The listing builds one solid part. Answer for the finished solid, in the listing's coordinates (mm). A direction names the side the tool comes from. Round coordinates to 2 decimals unless told otherwise and drop trailing zeros. Order: outer loops, then holes, each group sorted by start corner. A loop starts at its lowest first (then second) coordinate and runs counter-clockwise, first axis right, second up. Notation, with made-up numbers: M 63,70.5 L 100,70.5 A31 cw 100,109.5 Z; hole C 23.25,-1 d3. An arc over 180 degrees is marked long. Write item = value, one per line. Start each with the question number.
(1) For a pull along Z with two mould halves and no side action, classify faces 6 (the face through (-2, 58, -50)), 7 (the face through (-2.573, 119.082, -87.102)), 8 (the face through (-59.63, 23, 15)) as released by +Z, released by -Z, zero draft, split by the parting line, or undercut.
(2) Straight lines are drawn through the part: probe 1 along Z at (x, y) = (-1.5, 90.5); probe 2 along Y at (x, z) = (9, -2); probe 3 along X at (y, z) = (82, -42.5). For each, find the intervals that lie inside material, in ascending order. Write a range as from..to.
(3) Which of the six approach directions +Z, -Z, +X, -X, +Y, -Y give full straight-line access (tool end or side, diameter ignored) to faces 1 (the face through (-3, 43.505, 6)), 2 (the face through (17.87, 59, -34)), 3 (the face through (-2.57, 124, -80.01)), 4 (the face through (-33, 28, 0)), 5 (the face through (-2, 113.505, -80))?
(4) A cutting plane is placed at D-D, the plane x = 6. Determine the outline of the cut face in (y, z).
(5) Each of these flat-tipped pins is pushed along its axis until it touches: pin 1 (12 mm diameter, centred on x = 7, z = -63, fed in from +Y); pin 2 (8 mm diameter, centred on x = -1.05, z = -85.12, fed in from -Y); pin 3 (11 mm diameter, centred on x = -38.5, y = 28, fed in from -Z). Where does it stop, or does it pass through?
(6) A cutting plane is placed at C-C, the plane z = -98. Determine the outline of the cut face in (x, y).
(7) A cutting plane is placed at B-B, the plane y = 16.5. Determine the outline of the cut face in (x, z).
(8) A cutting plane is placed at A-A, the plane z = 12. Determine the outline of the cut face in (x, y), and give its area (3 significant figures).
from build123d import *

# Parameters (mm, degrees)
SKETCH2_W           = 115
SKETCH2_H           = 40
BOSS_EXTRUDE1_DEPTH = 60
CUT_EXTRUDE1_DEPTH  = 60
SKETCH4_R           = 10
CUT_EXTRUDE2_DEPTH  = 60
SKETCH5_W           = 40
SKETCH5_H           = 40
BOSS_EXTRUDE2_DEPTH = 50
SKETCH6_W           = 40
SKETCH6_H           = 20
BOSS_EXTRUDE3_DEPTH = 70
SKETCH7_W           = 40
SKETCH7_H           = 80
BOSS_EXTRUDE4_DEPTH = 10
SKETCH9_R           = 10
BOSS_EXTRUDE5_DEPTH = 1
SKETCH10_R          = 2.5
CUT_EXTRUDE3_DEPTH  = 15


with BuildPart() as part:
    # Sketch2 → Boss-Extrude1 (new body)
    with BuildSketch(Plane.XY):
        with Locations((-2.12962963, 23.505291005)):
            Rectangle(SKETCH2_W, SKETCH2_H)
    extrude(amount=BOSS_EXTRUDE1_DEPTH)

    # Sketch3 → Cut-Extrude1 (cut)
    with BuildSketch(Plane(origin=(0, 43.505291005, 0), x_dir=(1, 0, 0), z_dir=(0, 1, 0))):
        with BuildLine():
            Line((-59.62962963, -30), (-24.62962963, -30))
            ThreePointArc((-24.62962963, -30), (-2.12962963, -7.5), (20.37037037, -30))
            Line((20.37037037, -30), (55.37037037, -30))
            Line((55.37037037, -30), (55.37037037, -60))
            Line((55.37037037, -60), (-59.62962963, -60))
            Line((-59.62962963, -60), (-59.62962963, -30))
        make_face()
    extrude(amount=-CUT_EXTRUDE1_DEPTH, mode=Mode.SUBTRACT)

    # Sketch4 → Cut-Extrude2 (cut)
    with BuildSketch(Plane.XY.offset(30)):
        with Locations((-42.12962963, 23.505291005)):
            Circle(SKETCH4_R)
        with Locations((37.87037037, 23.505291005)):
            Circle(SKETCH4_R)
    extrude(amount=-CUT_EXTRUDE2_DEPTH, mode=Mode.SUBTRACT)

    # Sketch5 → Boss-Extrude2 (add)
    with BuildSketch(Plane(origin=(0, 0, 0), x_dir=(-1, 0, 0), z_dir=(0, 0, -1))):
        with Locations((2.12962963, 23.505291005)):
            Rectangle(SKETCH5_W, SKETCH5_H)
    extrude(amount=BOSS_EXTRUDE2_DEPTH)

    # Sketch6 → Boss-Extrude3 (add)
    with BuildSketch(Plane(origin=(0, 43.505291005, 0), x_dir=(1, 0, 0), z_dir=(0, 1, 0))):
        with Locations((-2.12962963, 40)):
            Rectangle(SKETCH6_W, SKETCH6_H)
    extrude(amount=BOSS_EXTRUDE3_DEPTH)

    # Sketch7 → Boss-Extrude4 (add)
    with BuildSketch(Plane(origin=(0, 113.505291005, 0), x_dir=(1, 0, 0), z_dir=(0, 1, 0))):
        with Locations((-2.12962963, 70)):
            Rectangle(SKETCH7_W, SKETCH7_H)
    extrude(amount=BOSS_EXTRUDE4_DEPTH)

    # Sketch9 → Boss-Extrude5 (add)
    with BuildSketch(Plane(origin=(0, 123.505291005, 0), x_dir=(1, 0, 0), z_dir=(0, 1, 0))):
        with Locations(Location((-2.12962963, 90, 0), (0, 0, 90))):
            Circle(SKETCH9_R)
    extrude(amount=BOSS_EXTRUDE5_DEPTH)

    # Sketch10 → Cut-Extrude3 (cut)
    with BuildSketch(Plane(origin=(0, 124.505291005, 0), x_dir=(1, 0, 0), z_dir=(0, 1, 0))):
        with Locations(Location((-6.896940429, 91.507563511, 0), (0, 0, 270))):
            Circle(SKETCH10_R)
        with Locations(Location((1.559614069, 93.374830505, 0), (0, 0, 270))):
            Circle(SKETCH10_R)
        with Locations(Location((-1.051562528, 85.117605984, 0), (0, 0, 270))):
            Circle(SKETCH10_R)
    extrude(amount=-CUT_EXTRUDE3_DEPTH, mode=Mode.SUBTRACT)


solid = part.part
Reported:
q1.face_6 = released by -Z
q1.face_7 = undercut
q1.face_8 = zero draft
q2.probe_1 = -50..-30
q2.probe_2 = 3.51..43.51
q2.probe_3 = -22.13..17.87
q3.face_1 = +Z, +X, -X, +Y
q3.face_2 = -Z, +X, +Y, -Y
q3.face_3 = +Y
q3.face_4 = -Z, -X, +Y, -Y
q3.face_5 = -Z, +X, -X, -Y
q4.outline = M 3.51,-50 L 113.51,-50 L 113.51,-110 L 123.51,-110 L 123.51,-95.82 L 124.51,-95.82 L 124.51,-84.18 L 123.51,-84.18 L 123.51,-30 L 43.51,-30 L 43.51,9.02 L 3.51,9.02 Z
q5.pin_1 = 123.51
q5.pin_2 = 113.51
q5.pin_3 = 0
q6.outline = M -22.13,113.51 L 17.87,113.51 L 17.87,123.51 L 3.87,123.51 L 3.87,124.51 L -8.13,124.51 L -8.13,123.51 L -22.13,123.51 Z
q7.outline = M -59.63,0 L -49.27,0 L -49.27,30 L -59.63,30 Z; M -34.99,0 L -22.13,0 L -22.13,-50 L 17.87,-50 L 17.87,0 L 30.73,0 L 30.73,30 L 20.37,30 A22.5 cw -24.63,30 L -34.99,30 Z; M 45.01,0 L 55.37,0 L 55.37,30 L 45.01,30 Z
q8.outline = M -59.63,3.51 L -15.63,3.51 L -15.63,43.51 L -59.63,43.51 Z; M 11.37,3.51 L 55.37,3.51 L 55.37,43.51 L 11.37,43.51 Z; hole C -42.13,23.51 d20; hole C 37.87,23.51 d20
q8.area = 2,890 mm²
